The listing builds one solid part. Answer for the finished solid, in the listing's coordinates (mm). Face numbers are marked on the shaded views. A direction names the side the tool comes from. Give positions to 0.01 mm unless a question says otherwise; leave off trailing zeros. Write each loop counter-clockwise with the first axis right and the second up, starting at its lowest first coordinate (ties: lowest second). Pieces come first, ordered by that corner, then holes. Notation, with made-up numbers: (53, 25) - (104, 25) arc R14 cw to (104, 45) - close; hole circle Ø3 at (5.5, -30). An arc over 180 degrees is marked (long way). Return JSON: item names as keys, results as strings.
from build123d import *

# Parameters (mm, degrees)
SALIENTE_EXTRUIR1_DEPTH = 10.72
CROQUIS2_R              = 0.775
SALIENTE_EXTRUIR2_DEPTH = 2.9
CHAFL_N1_SIZE           = 0.2
VACIADO1_START          = 0.61
VACIADO1_DEPTH          = 10.11
VACIADO1_START_2        = -2.29
VACIADO1_2_OUTLINE_R    = 0.165
VACIADO1_2_DEPTH        = 2.9
CROQUIS4_R              = 0.81
SALIENTE_EXTRUIR4_DEPTH = 9
REDONDEO1_R             = 0.7


# Read off the part's stored shape, not the designer's step: Vaciado1
with BuildPart() as part:
    # Croquis1 → Saliente-Extruir1 (new body)
    with BuildSketch(Plane.XY):
        with BuildLine():
            Line((-2.6, 7.63), (-2.6, 0))
            Line((-2.6, 0), (2.6, 0))
            Line((2.6, 0), (2.6, 7.63))
            ThreePointArc((2.6, 7.63), (0, 10.23), (-2.6, 7.63))
        make_face()
    extrude(amount=SALIENTE_EXTRUIR1_DEPTH)

    # Croquis2 → Saliente-Extruir2 (add)
    with BuildSketch(Plane(origin=(0, 0, 0), x_dir=(-1, 0, 0), z_dir=(0, 0, -1))):
        with Locations((0, 7.25)):
            Circle(CROQUIS2_R)
        with Locations((0, 2.25)):
            Circle(CROQUIS2_R)
    extrude(amount=SALIENTE_EXTRUIR2_DEPTH)

    # Chaflán1
    chafl_n1_edges = [part.edges().sort_by_distance(p)[0] for p in [
        (0.775, 7.25, -2.9),
        (0.775, 2.25, -2.9),
    ]]
    chamfer(chafl_n1_edges, length=CHAFL_N1_SIZE)

    # Vaciado1 outline → Vaciado1 (cut)
    with BuildSketch(Plane.XY.offset(VACIADO1_START)):
        with BuildLine():
            ThreePointArc((1.99, 7.63), (0, 9.62), (-1.99, 7.63))
            Line((-1.99, 7.63), (-1.99, 0.61))
            Line((-1.99, 0.61), (1.99, 0.61))
            Line((1.99, 0.61), (1.99, 7.63))
        make_face()
    extrude(amount=VACIADO1_DEPTH, mode=Mode.SUBTRACT)

    # Vaciado1 2 outline → Vaciado1 2 (cut)
    with BuildSketch(Plane.XY.offset(VACIADO1_START_2)):
        with Locations((0, 7.25)):
            Circle(VACIADO1_2_OUTLINE_R)
        with Locations((0, 2.25)):
            Circle(VACIADO1_2_OUTLINE_R)
    extrude(amount=VACIADO1_2_DEPTH, mode=Mode.SUBTRACT)

    # Croquis4 → Saliente-Extruir4 (add)
    with BuildSketch(Plane.XY.offset(0.61)):
        with Locations(Location((0, 2.25, 0), (0, 0, 180))):
            Circle(CROQUIS4_R)
        with Locations(Location((0, 7.25, 0), (0, 0, 180))):
            Circle(CROQUIS4_R)
    extrude(amount=SALIENTE_EXTRUIR4_DEPTH)

    # Redondeo1
    redondeo1_edges = [part.edges().sort_by_distance(p)[0] for p in [
        (0.81, 2.25, 9.61),
        (0.81, 7.25, 9.61),
    ]]
    fillet(redondeo1_edges, radius=REDONDEO1_R)


solid = part.part
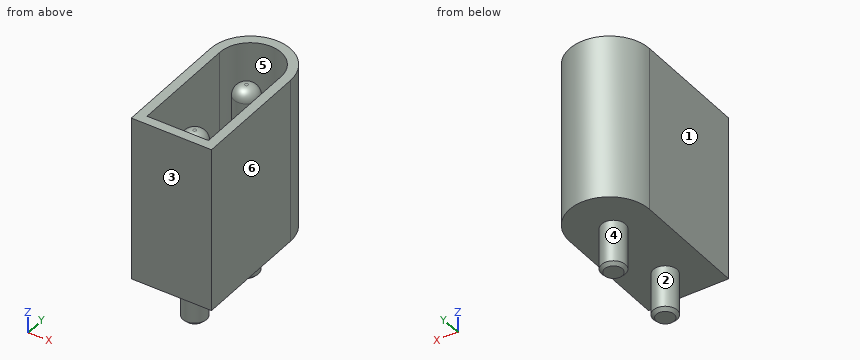
Item 1: A cutting plane is placed at A-A on z = 2. Determine the outline of the cut face in (x, y), then the cut area to 3 significant figures.
Answer below:
{"outline": "(-2.6, 0) - (2.6, 0) - (2.6, 7.63) arc R2.6 ccw to (-2.6, 7.63) - close; circle Ø1.62 at (0, 2.25); circle Ø1.62 at (0, 7.25); hole (-1.99, 0.61) - (1.99, 0.61) - (1.99, 7.63) arc R1.99 ccw to (-1.99, 7.63) - close", "area": "20.3 mm²"}
Item 2: The mould has two halves that part along Y. Classify the marked faces 1, 2 and 3: +Y half, -Y half, draft (parallel to the pull), parting line (faces both ways), or undercut.
Answer below:
{"face 1": "draft", "face 2": "undercut", "face 3": "-Y half"}
Item 3: A cutting plane is placed at D-D on x = 2.2. Determine the outline of the cut face in (y, z), then the cut area to 3 significant figures.
Answer below:
{"outline": "(0, 0) - (9.02, 0) - (9.02, 10.72) - (0, 10.72) - close", "area": "96.6 mm²"}
Item 4: A cutting plane is placed at B-B on y = 5.25. Determine the outline of the cut face in (x, z), then the cut area to 3 significant figures.
Answer below:
{"outline": "(-2.6, 0) - (2.6, 0) - (2.6, 10.72) - (1.99, 10.72) - (1.99, 0.61) - (-1.99, 0.61) - (-1.99, 10.72) - (-2.6, 10.72) - close", "area": "15.5 mm²"}
Item 5: For the marked faces 4, 5 and 6, determine the directions among +Z, -Z, +X, -X, +Y, -Y from which every point of the face is accessible in a straight line to the end or side of a thin tool.
Answer below:
{"face 4": "-Z", "face 5": "+Z", "face 6": "+Z, -Z, +X, +Y, -Y"}
Item 6: Flat-ended cylindrical pins translate along their axes: P1, Ø1.2, axis at x = 0.5, z = 5, coming from the +Y side; P2, Ø1, axis at x = 2, z = 5, coming from the +Y side. Find the tip coordinate at first contact, or state that the pin passes through.
Answer below:
{"P1": "stops at y = 10.23", "P2": "stops at y = 9.75"}
Item 7: Consider L1, parallel to Y at x = 0, z = -1.15 (3 decimals); L2, parallel to Y at x = -0.55, z = 1.75; L3, parallel to X at y = 5.5, z = 1. Determine where each line is inside the solid, lowest interval first.
Answer below:
{"L1": "y = 1.475 to 2.085, 2.415 to 3.025, 6.475 to 7.085, 7.415 to 8.025", "L2": "y = 0 to 0.61, 1.66 to 2.84, 6.66 to 7.84, 9.54 to 10.17", "L3": "x = -2.6 to -1.99, 1.99 to 2.6"}
Item 8: A cutting plane is placed at C-C on x = -1.35. Determine the outline of the cut face in (y, z), then the cut area to 3 significant figures.
Answer below:
{"outline": "(0, 0) - (9.85, 0) - (9.85, 10.72) - (9.09, 10.72) - (9.09, 0.61) - (0.61, 0.61) - (0.61, 10.72) - (0, 10.72) - close", "area": "19.9 mm²"}
